The model under review builds one solid part; all positions refer to its coordinate system, in mm. Round coordinates to 2 decimals unless told otherwise and drop trailing zeros. Write each loop counter-clockwise with the first axis right and the second up, starting at its lowest first coordinate (ties: lowest second). Pieces come first, ordered by that corner, then holes. Notation, with made-up numbers: (-35.75, 52) - (15.25, 52) arc R18 ccw to (15.25, 64) - close; hole circle Ø6 at (-19.75, -21). An arc over 180 degrees is marked (long way). One line per question, with ' | ' between items. Start each with the question number.
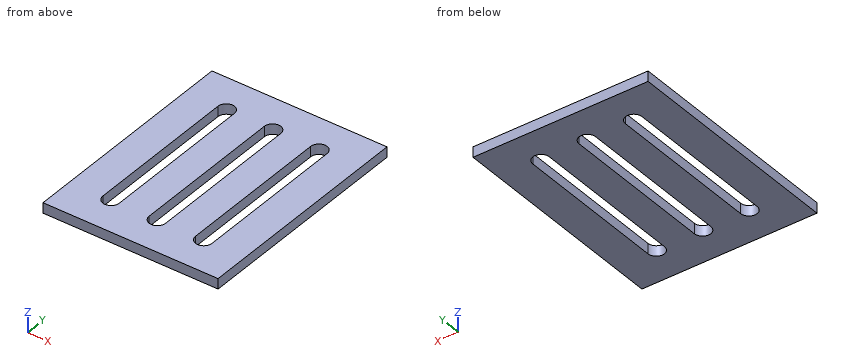
```python
from build123d import *

# Parameters (mm, degrees)
SKETCH3_W           = 170
SKETCH3_H           = 220
BOSS_EXTRUDE1_DEPTH = 5


with BuildPart() as part:
    # Sketch3 → Boss-Extrude1 (new, symmetric)
    with BuildSketch(Plane.XY):
        Rectangle(SKETCH3_W, SKETCH3_H)
        with BuildLine():
            Line((8, 75), (8, -75))
            ThreePointArc((8, -75), (0, -83), (-8, -75))
            Line((-8, -75), (-8, 75))
            ThreePointArc((-8, 75), (0, 83), (8, 75))
        make_face(mode=Mode.SUBTRACT)
        with BuildLine():
            Line((-37, 75), (-37, -75))
            ThreePointArc((-37, -75), (-45, -83), (-53, -75))
            Line((-53, -75), (-53, 75))
            ThreePointArc((-53, 75), (-45, 83), (-37, 75))
        make_face(mode=Mode.SUBTRACT)
        with BuildLine():
            Line((37, 75), (37, -75))
            ThreePointArc((37, -75), (45, -83), (53, -75))
            Line((53, -75), (53, 75))
            ThreePointArc((53, 75), (45, 83), (37, 75))
        make_face(mode=Mode.SUBTRACT)
    extrude(amount=BOSS_EXTRUDE1_DEPTH, both=True)


solid = part.part
```
1. Wall thickness on line 1 along X through (y, z) = (56.5, 3.5); line 2 along X through (y, z) = (-78.5, -1); line 3 along Y through (x, z) = (-40.5, -2.75): over which ranges is each line inside the solid? List them lowest first. Write a range as [from, to].
2. Add section A-A, the plane x = 0. Write out the cut boundary in (y, z).
3. Add section C-C, the plane z = 0.75. Write out the cut boundary in (x, y).
4. Add section B-B, the plane y = -68. Write out the cut boundary in (x, z), then the cut area to 3 significant figures.
Geometry check:
1) line 1: x = [-85, -53], [-37, -8], [8, 37], [53, 85] | line 2: x = [-85, -52.19], [-37.81, -7.19], [7.19, 37.81], [52.19, 85] | line 3: y = [-110, -81.61], [81.61, 110]
2) outline: (-110, -5) - (-83, -5) - (-83, 5) - (-110, 5) - close; (83, -5) - (110, -5) - (110, 5) - (83, 5) - close
3) outline: (-85, -110) - (85, -110) - (85, 110) - (-85, 110) - close; hole (-53, -75) arc R8 ccw to (-37, -75) - (-37, 75) arc R8 ccw to (-53, 75) - close; hole (-8, -75) arc R8 ccw to (8, -75) - (8, 75) arc R8 ccw to (-8, 75) - close; hole (37, -75) arc R8 ccw to (53, -75) - (53, 75) arc R8 ccw to (37, 75) - close
4) outline: (-85, -5) - (-53, -5) - (-53, 5) - (-85, 5) - close; (-37, -5) - (-8, -5) - (-8, 5) - (-37, 5) - close; (8, -5) - (37, -5) - (37, 5) - (8, 5) - close; (53, -5) - (85, -5) - (85, 5) - (53, 5) - close | area: 1,220 mm2
